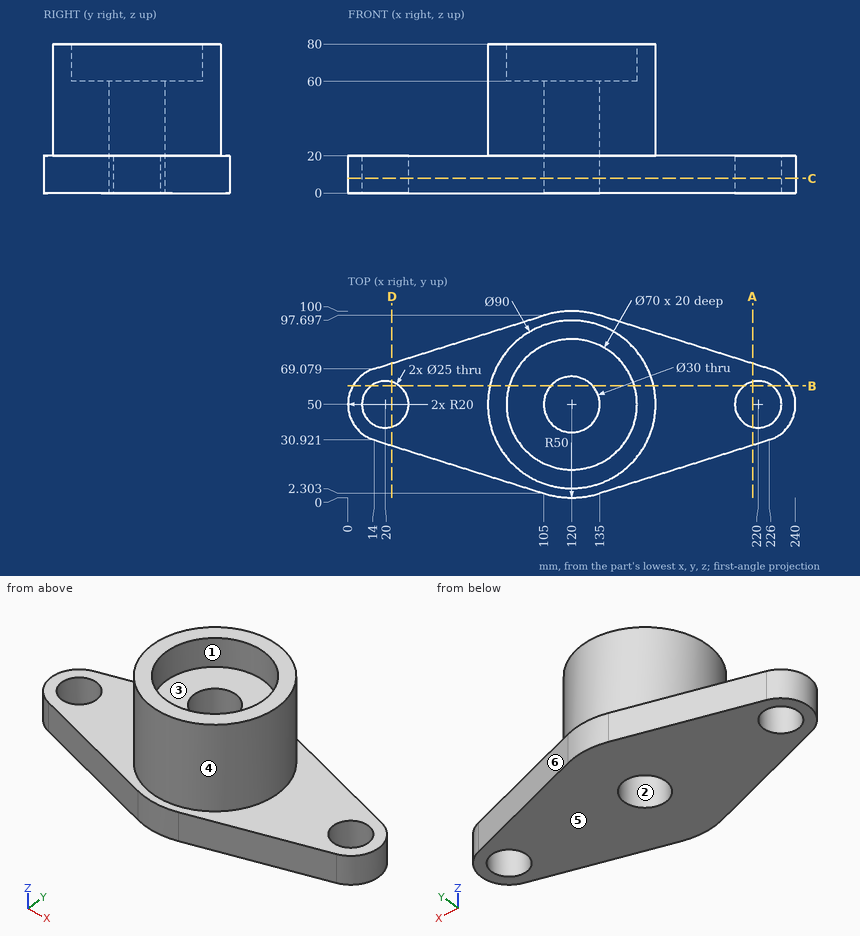
Job drawing, mm, ordinate dimensions from the low corner. One solid piece. A direction names the side the tool comes from. Give positions to 0.01 mm unless a question says otherwise; leave off trailing zeros. Loops run counter-clockwise (first coordinate to the right, second up) from the corner with the lowest first, then second, coordinate; pieces in that order, holes last. Notation, with made-up numbers: M -15.75,59.25 L 5.25,59.25 A24 ccw 5.25,72.25 Z; hole C -25,47 d5. An arc over 180 degrees is marked long. Return JSON: item names as keys, results as strings.
1) Saw through at D-D, the plane x = 23.5. List the corners of the cut face in (y, z).
Calculated:
{"outline": "M 27.93,0 L 38,0 L 38,20 L 27.93,20 Z; M 62,0 L 72.07,0 L 72.07,20 L 62,20 Z"}
2) Flat gauge pins, fed straight in: pin 1 Ø3 at (x, y) = (120, 68) entering from +Z; pin 2 Ø5 at (y, z) = (16.5, 23.5) entering from -X; pin 3 Ø2 at (y, z) = (58.5, 33) entering from +X. Where does each tip first touch, or does it go through?
Calculated:
{"pin 1": "stops at z = 60", "pin 2": "stops at x = 87.38", "pin 3": "stops at x = 164.37"}
3) Saw through at A-A, the plane x = 217. List the corners of the cut face in (y, z) (1 decimal), then the cut area to 3 significant figures.
Calculated:
{"outline": "M 28.1,0 L 37.9,0 L 37.9,20 L 28.1,20 Z; M 62.1,0 L 71.9,0 L 71.9,20 L 62.1,20 Z", "area": "391 mm2"}
4) 3-axis set-ups, long thin cutter, end or side, ignore diameter. For the marked faces 1 and 2: which of +Z, -Z, +X, -X, +Y, -Y reach the whole face in a straight line?
Calculated:
{"face 1": "+Z", "face 2": "+Z, -Z"}
5) Pull direction X, two halves, no side cores. Call the marked faces 3, 4, 5 and 6: released by +X, released by -X, zero draft, split by the parting line, or undercut.
Calculated:
{"face 3": "undercut", "face 4": "split by the parting line", "face 5": "zero draft", "face 6": "released by +X"}
6) Saw through at C-C, the plane z = 8. List the corners of the cut face in (x, y).
Calculated:
{"outline": "M 14,30.92 L 105,2.3 A50 ccw 135,2.3 L 226,30.92 A20 ccw 226,69.08 L 135,97.7 A50 ccw 105,97.7 L 14,69.08 A20 ccw Z; hole C 20,50 d25; hole C 120,50 d30; hole C 220,50 d25"}
7) Drill centre lines: line 1 (Z direction, x = 196, y = 28.5); line 2 (Z direction, x = 138, y = 36); line 3 (Y direction, x = 117.5, z = 56). Where is each one in solid material? Low to high.
Calculated:
{"line 1": "z = 0 to 20", "line 2": "z = 0 to 60", "line 3": "y = 5.07 to 35.21, 64.79 to 94.93"}
8) Saw through at B-B, the plane y = 60. List the corners of the cut face in (x, z) (1 decimal), then the cut area to 3 significant figures.
Calculated:
{"outline": "M 2.7,0 L 12.5,0 L 12.5,20 L 2.7,20 Z; M 27.5,0 L 108.8,0 L 108.8,60 L 86.5,60 L 86.5,80 L 76.1,80 L 76.1,20 L 27.5,20 Z; M 131.2,0 L 212.5,0 L 212.5,20 L 163.9,20 L 163.9,80 L 153.5,80 L 153.5,60 L 131.2,60 Z; M 227.5,0 L 237.3,0 L 237.3,20 L 227.5,20 Z", "area": "6,670 mm2"}
